```python
from build123d import *

# Parameters (mm, degrees)
SKETCH1_W           = 20.5
SKETCH1_H           = 20
BOSS_EXTRUDE1_DEPTH = 41
SKETCH3_W           = 20
SKETCH3_H           = 2.467931734
BOSS_EXTRUDE2_DEPTH = 10
SKETCH4_R           = 2.290313936
CUT_EXTRUDE9_DEPTH  = 10
SKETCH5_R           = 3.018718549
BOSS_EXTRUDE3_DEPTH = 12


with BuildPart() as part:
    # Sketch1 → Boss-Extrude1 (new body)
    with BuildSketch(Plane(origin=(0, 0, 0), x_dir=(1, 0, 0), z_dir=(0, 1, 0))):
        Rectangle(SKETCH1_W, SKETCH1_H)
    boss_extrude1 = extrude(amount=BOSS_EXTRUDE1_DEPTH)

    # Sketch3 → Boss-Extrude2 (add)
    with BuildSketch(Plane.ZY.offset(10.25)):
        with Locations((0, 32.759182637)):
            Rectangle(SKETCH3_W, SKETCH3_H)
    boss_extrude2 = extrude(amount=BOSS_EXTRUDE2_DEPTH)

    # Sketch4 → Cut-Extrude9 (cut)
    with BuildSketch(Plane(origin=(0, 33.993148504, 0), x_dir=(1, 0, 0), z_dir=(0, 1, 0))):
        with Locations(Location((-15.25, 5, 0), (0, 0, 270))):
            Circle(SKETCH4_R)
        with Locations(Location((-15.25, -5, 0), (0, 0, 270))):
            Circle(SKETCH4_R)
    cut_extrude9 = extrude(amount=-CUT_EXTRUDE9_DEPTH, mode=Mode.SUBTRACT)

    # Mirror1: Boss-Extrude1, Boss-Extrude2, Cut-Extrude9 across plane
    add(boss_extrude1.mirror(Plane(origin=(10.25, 41, -10), x_dir=(0, 0, 1), z_dir=(-1, 0, 0))))
    add(boss_extrude2.mirror(Plane(origin=(10.25, 41, -10), x_dir=(0, 0, 1), z_dir=(-1, 0, 0))))
    add(cut_extrude9.mirror(Plane(origin=(10.25, 41, -10), x_dir=(0, 0, 1), z_dir=(-1, 0, 0))), mode=Mode.SUBTRACT)

    # Sketch5 → Boss-Extrude3 (add)
    with BuildSketch(Plane(origin=(0, 41, 0), x_dir=(1, 0, 0), z_dir=(0, 1, 0))):
        with Locations(Location((20.5, 0, 0), (0, 0, 270))):
            Circle(SKETCH5_R)
    extrude(amount=BOSS_EXTRUDE3_DEPTH)


solid = part.part
```
Here's how the part is built. I have some questions about the finished solid (model axes, mm). A direction names the side the tool comes from. Coordinates: 2 decimals unless noted, no trailing zeros. Order: outer loops, then holes, each group sorted by start corner. A loop starts at its lowest first (then second) coordinate and runs counter-clockwise, first axis right, second up. Notation, with made-up numbers: (-20, 19.25) - (18, 19.25) arc R12 ccw to (18, 35.25) - close; hole circle Ø8 at (-26.75, 7.5). An arc over 180 degrees is marked (long way). One line per question, with ' | ' between items. Start each with the question number.
1. If we section it at A-A (z = -5): Write out the boundary of the cut face in (x, y).
2. Please list where these lines run through material, in increasing order: line 1 along X through (y, z) = (32.6, -5); line 2 along Z through (x, y) = (35.75, 32.6); line 3 along Z through (x, y) = (35, 33). Write a range as [from, to].
3. If we mould it in two halves opening along Z, with no side actions, what happens to faces 1 (the flat face through (-15, 33.993, 0)), 2 (the cylindrical face through (37.986, 32.776, 4.504)), 3 (the flat face through (11, 20, 10))? For each: released by +Z, released by -Z, zero draft, split by the parting line, or undercut.
4. If we section it at D-D (x = 20.5): Write out the boundary of the cut face in (y, z).
5. If we section it at B-B (x = -15.25): Write out the boundary of the cut face in (y, z), and give its area (3 significant figures).
6. I'm going to push flat-ended pins straight in: pin 1 Ø6 at (x, z) = (-15.25, 5) entering from -Y; pin 2 Ø4 at (x, z) = (8.5, 4.5) entering from +Y; pin 3 Ø2 at (y, z) = (37, -1) entering from -X; pin 4 Ø8 at (y, z) = (36, 0.5) entering from -X. Where does each tip first touch, or does it pass through?
7. If we section it at C-C (z = 0): Write out the boundary of the cut face in (x, y), and give its area (3 significant figures).
8. Which directions (+Z, -Z, +X, -X, +Y, -Y) give clear straight access to the entire face, cutting with the end or side of a thin tool? Please do faces 4 (the cylindrical face through (23.493, 46.916, -0.393)), 5 (the flat face through (-15, 31.525, 0)), 6 (the flat face through (36, 33.993, 0)), 7 (the flat face through (36, 31.525, 0)), 8 (the flat face through (-10.25, 37, 0)).
Model answer:
1) outline: (-20.25, 31.53) - (-17.54, 31.53) - (-17.54, 33.99) - (-20.25, 33.99) - close; (-12.96, 31.53) - (-10.25, 31.53) - (-10.25, 0) - (30.75, 0) - (30.75, 31.53) - (33.46, 31.53) - (33.46, 33.99) - (30.75, 33.99) - (30.75, 41) - (-10.25, 41) - (-10.25, 33.99) - (-12.96, 33.99) - close; (38.04, 31.53) - (40.75, 31.53) - (40.75, 33.99) - (38.04, 33.99) - close
2) line 1: x = [-20.25, -17.54], [-12.96, 33.46], [38.04, 40.75] | line 2: z = [-10, -7.29], [-2.71, 2.71], [7.29, 10] | line 3: z = [-10, -7.16], [-2.84, 2.84], [7.16, 10]
3) face 1: zero draft | face 2: undercut | face 3: released by +Z
4) outline: (0, -10) - (41, -10) - (41, -3.02) - (53, -3.02) - (53, 3.02) - (41, 3.02) - (41, 10) - (0, 10) - close
5) outline: (31.53, -10) - (33.99, -10) - (33.99, -7.29) - (31.53, -7.29) - close; (31.53, -2.71) - (33.99, -2.71) - (33.99, 2.71) - (31.53, 2.71) - close; (31.53, 7.29) - (33.99, 7.29) - (33.99, 10) - (31.53, 10) - close | area: 26.7 mm²
6) pin 1: stops at y = 31.53 | pin 2: stops at y = 41 | pin 3: stops at x = -10.25 | pin 4: stops at x = -20.25
7) outline: (-20.25, 31.53) - (-10.25, 31.53) - (-10.25, 0) - (30.75, 0) - (30.75, 31.53) - (40.75, 31.53) - (40.75, 33.99) - (30.75, 33.99) - (30.75, 41) - (23.52, 41) - (23.52, 53) - (17.48, 53) - (17.48, 41) - (-10.25, 41) - (-10.25, 33.99) - (-20.25, 33.99) - close | area: 1,800 mm²
8) face 4: +Y | face 5: +Z, -Z, -X, -Y | face 6: +Z, -Z, +X, +Y | face 7: +Z, -Z, +X, -Y | face 8: +Z, -Z, -X, +Y
